Geometry check sheet. Reference: the model listing, model coordinates, mm. A direction names the side the tool comes from. Give positions to 0.01 mm unless a question says otherwise; leave off trailing zeros. Order: outer loops, then holes, each group sorted by start corner. A loop starts at its lowest first (then second) coordinate and runs counter-clockwise, first axis right, second up.
from build123d import *

# Parameters (mm, degrees)
SKETCH1_W           = 90
SKETCH1_H           = 35
SKETCH1_R           = 5.5
SKETCH1_R_2         = 1.5
SKETCH1_R_3         = 11
BOSS_EXTRUDE1_DEPTH = 6
SKETCH2_W           = 90
SKETCH2_H           = 3
BOSS_EXTRUDE2_DEPTH = 20
SKETCH4_R           = 2.5
CUT_EXTRUDE1_DEPTH  = 10
SKETCH5_R           = 2.7
CUT_EXTRUDE2_DEPTH  = 10


with BuildPart() as part:
    # Sketch1 → Boss-Extrude1 (new body)
    with BuildSketch(Plane.XY):
        Rectangle(SKETCH1_W, SKETCH1_H)
        with Locations((-30, 0)):
            Circle(SKETCH1_R, mode=Mode.SUBTRACT)
        with Locations((-38, 0)):
            Circle(SKETCH1_R_2, mode=Mode.SUBTRACT)
        with Locations((-22, 0)):
            Circle(SKETCH1_R_2, mode=Mode.SUBTRACT)
        with Locations((29.999666666, 0.2)):
            Circle(SKETCH1_R_3, mode=Mode.SUBTRACT)
    extrude(amount=BOSS_EXTRUDE1_DEPTH)

    # Sketch2 → Boss-Extrude2 (add)
    with BuildSketch(Plane.XY.offset(6)):
        with Locations((0, -16)):
            Rectangle(SKETCH2_W, SKETCH2_H)
    extrude(amount=BOSS_EXTRUDE2_DEPTH)

    # Sketch4 → Cut-Extrude1 (cut)
    with BuildSketch(Plane.XY.offset(6)):
        with Locations((15, -7.5)):
            Circle(SKETCH4_R)
        with Locations(Location((-15, -7.5, 0), (0, 0, 180))):
            Circle(SKETCH4_R)
        with BuildLine():
            Line((2.5, 9.778989608), (2.5, 0.141519694))
            ThreePointArc((2.5, 0.141519694), (0, -2.358480306), (-2.5, 0.141519694))
            Line((-2.5, 0.141519694), (-2.5, 9.778989608))
            ThreePointArc((-2.5, 9.778989608), (0, 12.278989608), (2.5, 9.778989608))
        make_face()
    extrude(amount=-CUT_EXTRUDE1_DEPTH, mode=Mode.SUBTRACT)

    # Sketch5 → Cut-Extrude2 (cut)
    with BuildSketch(Plane(origin=(0, -14.5, 0), x_dir=(1, 0, 0), z_dir=(0, 1, 0))):
        with Locations(Location((30, -18.5, 0), (0, 0, 270))):
            Circle(SKETCH5_R)
        with Locations(Location((-30, -18.5, 0), (0, 0, 270))):
            Circle(SKETCH5_R)
    extrude(amount=-CUT_EXTRUDE2_DEPTH, mode=Mode.SUBTRACT)


solid = part.part
Item 1: Scan lines: L1, parallel to Y at x = -30, z = 1.8; L2, parallel to Y at x = 15, z = 1.6; L3, parallel to Y at x = 41, z = 24.5. Record each from-to range of solid material in increasing order.
Reported:
L1: y = -17.5 to -5.5, 5.5 to 17.5
L2: y = -17.5 to -10, -5 to 17.5
L3: y = -17.5 to -14.5
Item 2: Set-up check for faces 4 (the flat face through (-11, 2, 6)), 5 (the flat face through (-2.5, 5, 3)), 6 (the flat face through (-1, -17.5, 13)): record each of +Z, -Z, +X, -X, +Y, -Y from which the full face is reachable in a straight line by a thin tool's end or side.
Reported:
face 4: +Z, +X, -X, +Y
face 5: +Z, -Z
face 6: +Z, -Z, +X, -X, -Y
Item 3: Draft check along X on faces 1 (the flat face through (45, -4, 5)), 2 (the cylindrical face through (-39.2, -0.9, 3)), 3 (the flat face through (-1, -14.5, 16)). Enter one of: released by +X, released by -X, zero draft, split by the parting line, or undercut.
Reported:
face 1: released by +X
face 2: undercut
face 3: zero draft
Item 4: Sectioned sample at A-A (x = -22). Enter the section's corners in (y, z).
Reported:
outline: (-17.5, 0) - (-1.5, 0) - (-1.5, 6) - (-14.5, 6) - (-14.5, 26) - (-17.5, 26) - close; (1.5, 0) - (17.5, 0) - (17.5, 6) - (1.5, 6) - close
Item 5: Sectioned sample at D-D (y = -7.5). Enter the section's corners in (x, z), and give its area (3 significant figures).
Reported:
outline: (-45, 0) - (-17.5, 0) - (-17.5, 6) - (-45, 6) - close; (-12.5, 0) - (12.5, 0) - (12.5, 6) - (-12.5, 6) - close; (17.5, 0) - (22.14, 0) - (22.14, 6) - (17.5, 6) - close; (37.86, 0) - (45, 0) - (45, 6) - (37.86, 6) - close
area: 386 mm2
Item 6: Gauge pin test, flat ends, axial feed: pin 1 (7 mm diameter, centred on x = 30, z = 18.5, fed in from +Y); pin 2 (6.5 mm diameter, centred on x = 15, y = -7.5, fed in from -Z); pin 3 (4.5 mm diameter, centred on x = -30, z = 18.5, fed in from +Y); pin 4 (4 mm diameter, centred on x = -17.5, y = -4, fed in from +Z). Record the tip position at first contact, or that the pin passes through.
Reported:
pin 1: stops at y = -14.5
pin 2: stops at z = 0
pin 3: passes through
pin 4: stops at z = 6
Item 7: Sectioned sample at C-C (z = 20). Enter the section's corners in (x, y) (3 decimals).
Reported:
outline: (-45, -17.5) - (-32.245, -17.5) - (-32.245, -14.5) - (-45, -14.5) - close; (-27.755, -17.5) - (27.755, -17.5) - (27.755, -14.5) - (-27.755, -14.5) - close; (32.245, -17.5) - (45, -17.5) - (45, -14.5) - (32.245, -14.5) - close
Item 8: Sectioned sample at B-B (z = 2.25). Enter the section's corners in (x, y), and give its area (3 significant figures).
Reported:
outline: (-45, -17.5) - (45, -17.5) - (45, 17.5) - (-45, 17.5) - close; hole circle Ø3 at (-38, 0); hole circle Ø11 at (-30, 0); hole circle Ø3 at (-22, 0); hole circle Ø5 at (-15, -7.5); hole (-2.5, 0.14) arc R2.5 ccw to (2.5, 0.14) - (2.5, 9.78) arc R2.5 ccw to (-2.5, 9.78) - close; hole circle Ø5 at (15, -7.5); hole circle Ø22 at (30, 0.2)
area: 2,550 mm2
